Job drawing, mm, ordinate dimensions from the low corner. One solid piece. Round coordinates to 2 decimals unless told otherwise and drop trailing zeros. Order: outer loops, then holes, each group sorted by start corner. A loop starts at its lowest first (then second) coordinate and runs counter-clockwise, first axis right, second up. Notation, with made-up numbers: (56.5, 5.5) -> (70.5, 5.5) arc R32 cw to (70.5, 35.5) -> close; hole circle Ø6 at (39.5, 39). An arc over 180 degrees is marked (long way). Return JSON: item names as keys, results as strings. Group by question number.
Q1. Flat gauge pins, fed straight in: pin 1 (1.5 mm diameter, centred on x = 198, y = 3.5, fed in from +Z); pin 2 (1.5 mm diameter, centred on x = 196.5, y = 1.5, fed in from -Z); pin 3 (2.5 mm diameter, centred on y = 2.5, z = 67, fed in from +X). Where does each tip first touch, or does it go through?
Q2. Probe line 1 along X through (y, z) = (4.3, 140). List the from-to ranges inside material, lowest first.
Q3. Cut at B-B (z = 136.5). Write the cut outline in (x, y), then the cut area to 3 significant figures.
Q4. Cut at A-A (y = 4.25). Write the cut outline in (x, z), then the cut area to 3 significant figures.
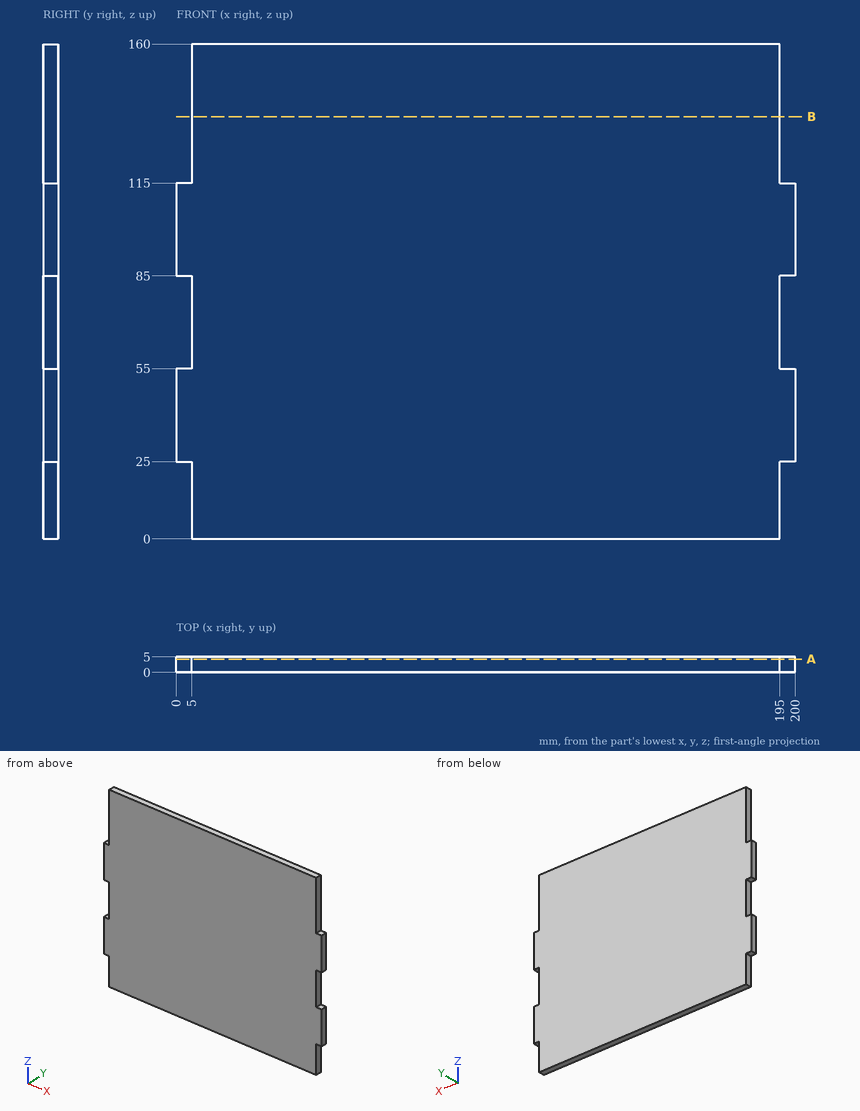
Solution:
{
 "1": {"pin 1": "stops at z = 115", "pin 2": "stops at z = 25", "pin 3": "stops at x = 195"},
 "2": {"line 1": "x = 5 to 195"},
 "3": {"outline": "(5, 0) -> (195, 0) -> (195, 5) -> (5, 5) -> close", "area": "950 mm²"},
 "4": {"outline": "(0, 25) -> (5, 25) -> (5, 0) -> (195, 0) -> (195, 25) -> (200, 25) -> (200, 55) -> (195, 55) -> (195, 85) -> (200, 85) -> (200, 115) -> (195, 115) -> (195, 160) -> (5, 160) -> (5, 115) -> (0, 115) -> (0, 85) -> (5, 85) -> (5, 55) -> (0, 55) -> close", "area": "31,000 mm²"}
}
